from build123d import *

# Parameters (mm, degrees)
F0_R      = 34.5568436117
F0_R_2    = 24.3288327677
F1_DEPTH  = 50.8
F2_W      = 74.3876788765
F2_H      = 46.9968635589
F3_DEPTH  = 25.4
F4_DEPTH  = 19.05
F5_DEPTH  = 19.05
F6_DEPTH  = 50.8
F7_W      = 10.3796771728
F7_H      = 25.9491894394
F8_DEPTH  = 50.8
F10_DEPTH = 76.2


with BuildPart() as f1:
    # F0 (on Top) → F1 (new body)
    with BuildSketch(Plane.XY):
        with Locations((33.8781066239, 0)):
            Circle(F0_R)
        with Locations((33.8781066239, 0)):
            Circle(F0_R_2, mode=Mode.SUBTRACT)
    extrude(amount=F1_DEPTH)

    # F2 (on Top) → F3 (join)
    with BuildSketch(Plane.XY):
        with Locations((-22.9217847809, -1.8741087988)):
            Rectangle(F2_W, F2_H)
    extrude(amount=F3_DEPTH)

    # F4 (cut): a face of the model
    f4_faces = [f1.faces().sort_by_distance(p)[0] for p in [
        (0.2986781504, 0, 50.8),
    ]]
    extrude(f4_faces, amount=-F4_DEPTH, mode=Mode.SUBTRACT)

    # F5 (cut): a face of the model
    f5_faces = [f1.faces().sort_by_distance(p)[0] for p in [
        (-28.8538449791, -2.0648821255, 25.4),
    ]]
    extrude(f5_faces, amount=-F5_DEPTH, mode=Mode.SUBTRACT)

    # F6 (cut): a face of the model
    f6_faces = [f1.faces().sort_by_distance(p)[0] for p in [
        (12.3662875308, 0, 25.4),
    ]]
    extrude(f6_faces, amount=-F6_DEPTH, mode=Mode.SUBTRACT)

    # F7 (on Right) → F8 (join)
    with BuildSketch(Plane.YZ):
        with Locations((-0.4324859474, 18.7410814688)):
            Rectangle(F7_W, F7_H)
    extrude(amount=-F8_DEPTH)

    # F9 (on face) → F10 (cut)
    with BuildSketch(Plane.XZ.offset(5.6223245338)):
        Polygon((-50.8, 6.35), (-0.2182994512, 31.7156761885), (-50.8, 31.7156761885), align=None)
    extrude(amount=-F10_DEPTH, mode=Mode.SUBTRACT)


solid = f1.part
Geometry: final body of the model. Coordinates: model frame, mm. A direction names the side the tool comes from. Coordinates: 2 decimals unless noted, no trailing zeros. Write each loop counter-clockwise with the first axis right and the second up, starting at its lowest first coordinate (ties: lowest second). Pieces come first, ordered by that corner, then holes. Notation, with made-up numbers: (37, 69.25) - (74, 69.25) arc R33 cw to (74, 99.25) - close; hole circle Ø7 at (-15.5, -29.75). An arc over 180 degrees is marked (long way). Return JSON: item names as keys, results as strings.
Item 1: Section query B-B (x = 54.5). Output: boundary loops of the cut face in (y, z).
Completed:
{"outline": "(-27.73, 0) - (-12.91, 0) - (-12.91, 31.75) - (-27.73, 31.75) - close; (12.91, 0) - (27.73, 0) - (27.73, 31.75) - (12.91, 31.75) - close"}
Item 2: Pin query (flat end, axial travel): pin 1 Ø12.5 at (x, z) = (-20, 19) entering from -Y; pin 2 Ø7 at (x, z) = (-14, 1.5) entering from -Y; pin 3 Ø5 at (y, z) = (15.5, 19.5) entering from -X; pin 4 Ø10 at (x, y) = (-29.5, -10.5) entering from -Z. Return the tip coordinate at first contact, or that it passes through.
Completed:
{"pin 1": "stops at y = -5.62", "pin 2": "stops at y = -25.37", "pin 3": "stops at x = 1.86", "pin 4": "stops at z = 0"}
Item 3: Line query: L1, parallel to Y at x = 12.5, z = 18; L2, parallel to Z at x = -37, y = -20.5; L3, parallel to X at y = -15, z = 16.5. Output: solid intervals per line, ascending.
Completed:
{"L1": "y = -27.15 to -11.61, 11.61 to 27.15", "L2": "z = 0 to 6.35", "L3": "x = 2.75 to 14.72, 53.03 to 65.01"}
Item 4: Section query D-D (y = -17). Output: boundary loops of the cut face in (x, z).
Completed:
{"outline": "(-60.12, 0) - (16.47, 0) - (16.47, 31.75) - (3.79, 31.75) - (3.79, 6.35) - (-60.12, 6.35) - close; (51.28, 0) - (63.96, 0) - (63.96, 31.75) - (51.28, 31.75) - close"}
Item 5: Section query C-C (z = 28.5). Output: boundary loops of the cut face in (x, y), and give its area (3 significant figures).
Completed:
{"outline": "(-6.63, -5.62) - (-0.22, -5.62) arc R34.56 ccw (long way) to (-0.35, 4.76) - (-6.63, 4.76) - close; hole circle Ø48.66 at (33.88, 0)", "area": "1,960 mm2"}
Item 6: Pull-direction query (X, two-part tool) for faces 5 (the face through (66.84, 10.38, 15.65)), 6 (the face through (57.083, 7.308, 15.653)), 7 (the face through (-25, -25.373, 3)), 8 (the face through (-25.863, -1.328, 18.855)); classes: +X half, -X half, draft (parallel to the pull), parting line (faces both ways), or undercut.
Completed:
{"face 5": "parting line", "face 6": "undercut", "face 7": "draft", "face 8": "-X half"}
Item 7: Reachability of faces 1 (the face through (-33, -7, 6.35)), 2 (the face through (-27, 21.624, 3)), 3 (the face through (-20, 4.757, 16)), 4 (the face through (-20, -5.622, 16)) from +Z, -Z, +X, -X, +Y, -Y: full face, straight path, thin tool, end or side. Return the list, or none.
Completed:
{"face 1": "+Z, -X", "face 2": "+Z, -Z, -X, +Y", "face 3": "+Z, -X, +Y", "face 4": "+Z, -X, -Y"}
